Here's how the part is built. I have some questions about the finished solid (model axes, mm). A direction names the side the tool comes from. Round coordinates to 2 decimals unless told otherwise and drop trailing zeros. Loops run counter-clockwise (first coordinate to the right, second up) from the corner with the lowest first, then second, coordinate; pieces in that order, holes last. Notation, with made-up numbers: (52, 50) - (69, 50) arc R30 cw to (69, 72) - close; hole circle Ø10 at (10, -19.75). An arc over 180 degrees is marked (long way). Return JSON: item names as keys, results as strings. Group by question number.
```python
from build123d import *

# Parameters (mm, degrees)
SKETCH1_W               = 22.054431489
SKETCH1_H               = 12.5
BOSS_EXTRUDE1_DEPTH     = 38
CUT_EXTRUDE1_DEPTH      = 10
CUT_EXTRUDE1_DEPTH_BACK = 15
SKETCH2_R               = 1.5
FILLET3_R               = 2
SKETCH5_R               = 1.5
CUT_EXTRUDE4_DEPTH      = 53.86644408
SKETCH16_W              = 22.05443149
SKETCH16_H              = 2.749314183
SKETCH16_W_2            = 22.143232671
SKETCH16_H_2            = 2.765172048
CUT_EXTRUDE6_DEPTH      = 8.5
FILLET4_R               = 2
SKETCH17_W              = 18.547612126
SKETCH17_H              = 2.749314183
SKETCH17_H_2            = 2.765172048
CUT_EXTRUDE7_DEPTH      = 5
SKETCH18_W              = 23.880033653
SKETCH18_H              = 0.742090051
SKETCH18_W_2            = 23.982039935
SKETCH18_H_2            = 0.706785536
CUT_EXTRUDE8_DEPTH      = 20


with BuildPart() as part:
    # Sketch1 → Boss-Extrude1 (new body)
    with BuildSketch(Plane.XY):
        with Locations((-13.228930986, -24.070183414)):
            Rectangle(SKETCH1_W, SKETCH1_H)
    extrude(amount=BOSS_EXTRUDE1_DEPTH)

    # Sketch2 → Cut-Extrude1 (cut, two sides: drawn at the far end of the back side and taken through both)
    with BuildSketch(Plane.XZ.offset(30.320183414).offset(-CUT_EXTRUDE1_DEPTH_BACK)):
        with Locations(Location((-13.228930986, 6.5, 0), (0, 0, 90))):
            Circle(SKETCH2_R)
        with Locations(Location((-13.228930986, 31.5, 0), (0, 0, 90))):
            Circle(SKETCH2_R)
        with BuildLine():
            Line((-4.478930986, 29.25), (-2.201715242, 29.25))
            add(Edge.make_bspline(
                [(-24.256146731, 29.25), (-34.277912729, 38.417119108), (-13.227499763, 50.308047167), (7.840407292, 38.416977249), (-2.201715242, 29.25)],
                knots=[0, 0, 0, 0, 0.49986218, 1, 1, 1, 1], degree=3))
            add(Edge.make_bspline(
                [(-6.103895584, 34.329012749), (-10.720559386, 33.527203043), (-28.641384523, 40.845191705), (-24.256146731, 29.25)],
                knots=[0, 0, 0, 0, 1, 1, 1, 1], degree=3))
            ThreePointArc((-6.103895584, 34.329012749), (-4.895067543, 31.916312081), (-4.478930986, 29.25))
        make_face()
        with BuildLine():
            Line((-4.478930986, 8.75), (-2.201715242, 8.75))
            add(Edge.make_bspline(
                [(-2.201715242, 8.75), (5.39210746, 3.880294823), (-0.777052631, -4.523329032), (-17.174300591, -10.623347238), (-34.821400648, -0.026005424), (-24.256146731, 8.75)],
                knots=[0, 0, 0, 0, 0.283272691, 0.504244858, 1, 1, 1, 1], degree=3))
            add(Edge.make_bspline(
                [(-23.490579314, 0), (-24.966512963, 4.237786421), (-24.256146731, 8.75)],
                knots=[0, 0, 0, 1, 1, 1], degree=2))
            Line((-23.490579314, 0), (-13.228930986, 0))
            ThreePointArc((-13.228930986, 0), (-7.041746651, 2.562815665), (-4.478930986, 8.75))
        make_face()
    extrude(amount=CUT_EXTRUDE1_DEPTH + CUT_EXTRUDE1_DEPTH_BACK, mode=Mode.SUBTRACT)

    # Fillet3
    # the kernel refuses this fillet: 2 mm, written as the material it takes off along each edge
    with BuildSketch(Plane(origin=(-24.256146731, -17.820183414, -5.498495188), x_dir=(1, 0, 0), z_dir=(0, 0, 1))) as fillet3_piece_1:
        with BuildLine():
            CenterArc((FILLET3_R, -FILLET3_R), FILLET3_R, 90, 90)
            Line((0, -FILLET3_R), (-FILLET3_R * 0.02, -FILLET3_R))
            Line((-FILLET3_R * 0.02, -FILLET3_R), (-FILLET3_R * 0.02, FILLET3_R * 0.02))
            Line((-FILLET3_R * 0.02, FILLET3_R * 0.02), (FILLET3_R, FILLET3_R * 0.02))
            Line((FILLET3_R, FILLET3_R * 0.02), (FILLET3_R, 0))
        make_face()
    extrude(amount=44.984872581, mode=Mode.SUBTRACT)
    with BuildSketch(Plane(origin=(-24.256146731, -30.320183414, -5.498495188), x_dir=(1, 0, 0), z_dir=(0, 0, 1))) as fillet3_piece_2:
        with BuildLine():
            CenterArc((FILLET3_R, FILLET3_R), FILLET3_R, 180, 90)
            Line((0, FILLET3_R), (-FILLET3_R * 0.02, FILLET3_R))
            Line((-FILLET3_R * 0.02, FILLET3_R), (-FILLET3_R * 0.02, -FILLET3_R * 0.02))
            Line((-FILLET3_R * 0.02, -FILLET3_R * 0.02), (FILLET3_R, -FILLET3_R * 0.02))
            Line((FILLET3_R, -FILLET3_R * 0.02), (FILLET3_R, 0))
        make_face()
    extrude(amount=44.984872581, mode=Mode.SUBTRACT)
    with BuildSketch(Plane(origin=(-24.256146731, -17.374523396, 3.001504812), x_dir=(0.16676818592575765, -1.261066300243152e-15, -0.9859961319209278), z_dir=(0, -1, 0))) as fillet3_piece_3:
        with BuildLine():
            CenterArc((0.168096911, 1.999974157), FILLET3_R, 260.400032587, 9.891234523)
            Line((-0.165439461, 0.027981894), (-0.172110188, -0.011457952))
            Line((-0.172110188, -0.011457952), (-0.006670727, -0.039439845))
            Line((-0.006670727, -0.039439845), (-0.00020343, -0.039999483))
            ThreePointArc((-0.00020343, -0.039999483), (0.089132026, -0.040226606), (0.178467349, -0.039999483))
            Line((0.178467349, -0.039999483), (0.178264007, 0))
        make_face()
    extrude(amount=13.391320036, mode=Mode.SUBTRACT)
    with BuildSketch(Plane(origin=(-24.256146731, -14.125185169, 34.486377393), x_dir=(0.8125654725305003, 0, 0.5828699279009725), z_dir=(0, -1, 0))) as fillet3_piece_4:
        with BuildLine():
            CenterArc((1.058597408, -1.955531144), FILLET3_R, 77.895172565, 66.452175148)
            Line((-0.566533537, -0.789791288), (-0.599036156, -0.766476491))
            Line((-0.599036156, -0.766476491), (-0.032502619, 0.023314797))
            Line((-0.032502619, 0.023314797), (-0.009827922, 0.038773856))
            ThreePointArc((-0.009827922, 0.038773856), (0.740246051, 0.125750941), (1.486387336, 0.039110623))
            Line((1.486387336, 0.039110623), (1.477999298, 0))
        make_face()
    extrude(amount=19.88999649, mode=Mode.SUBTRACT)

    # Sketch5 → Cut-Extrude4 (cut, through all)
    with BuildSketch(Plane.XY):
        with Locations(Location((-18.011106811, -24.070183414, 0), (0, 0, 180))):
            Circle(SKETCH5_R)
        with Locations(Location((-8.446755162, -24.070183414, 0), (0, 0, 180))):
            Circle(SKETCH5_R)
    extrude(amount=CUT_EXTRUDE4_DEPTH, mode=Mode.SUBTRACT)

    # Sketch16 → Cut-Extrude6 (cut)
    with BuildSketch(Plane.XY.offset(38)):
        with Locations((-13.228930985, -20.306320009)):
            Rectangle(SKETCH16_W, SKETCH16_H)
        with Locations((-13.184530395, -27.841975748)):
            Rectangle(SKETCH16_W_2, SKETCH16_H_2)
    extrude(amount=-CUT_EXTRUDE6_DEPTH, mode=Mode.SUBTRACT)

    # Fillet4
    # the kernel refuses this fillet: 2 mm, written as the material it takes off along each edge
    with BuildSketch(Plane(origin=(-6.103895584, -22.334365667, 34.329012749), x_dir=(0.515368054600745, 0, -0.8569689424343473), z_dir=(0, 1, 0))) as fillet4_piece_1:
        with BuildLine():
            CenterArc((1.205528974, 1.993941708), FILLET4_R, 212.228268917, 62.232476225)
            Line((-0.486331325, 0.927354287), (-0.520168531, 0.906022538))
            ThreePointArc((-0.520168531, 0.906022538), (-0.25689069, 0.456334761), (-0.037300681, -0.01444504))
            Line((-0.037300681, -0.01444504), (-0.003111043, -0.039878834))
            ThreePointArc((-0.003111043, -0.039878834), (0.68054055, -0.066505026), (1.364192143, -0.039878834))
            Line((1.364192143, -0.039878834), (1.3610811, 0))
        make_face()
    extrude(amount=7.916885004, mode=Mode.SUBTRACT)
    with BuildSketch(Plane(origin=(-6.103895584, -29.862092474, 34.329012749), x_dir=(0.515368054600745, 0, -0.8569689424343473), z_dir=(0, 1, 0))) as fillet4_piece_2:
        with BuildLine():
            CenterArc((1.205528974, 1.993941708), FILLET4_R, 212.228268917, 62.232476225)
            Line((-0.486331325, 0.927354287), (-0.520168531, 0.906022538))
            ThreePointArc((-0.520168531, 0.906022538), (-0.25689069, 0.456334761), (-0.037300681, -0.01444504))
            Line((-0.037300681, -0.01444504), (-0.003111043, -0.039878834))
            ThreePointArc((-0.003111043, -0.039878834), (0.68054055, -0.066505026), (1.364192143, -0.039878834))
            Line((1.364192143, -0.039878834), (1.3610811, 0))
        make_face()
    extrude(amount=11.583818124, mode=Mode.SUBTRACT)
    with BuildSketch(Plane(origin=(-6.103895584, -33.722886164, 34.329012749), x_dir=(0.515368054600745, 0, -0.8569689424343473), z_dir=(0, 1, 0))) as fillet4_piece_3:
        with BuildLine():
            CenterArc((1.205528974, 1.993941708), FILLET4_R, 212.228268917, 62.232476225)
            Line((-0.486331325, 0.927354287), (-0.520168531, 0.906022538))
            ThreePointArc((-0.520168531, 0.906022538), (-0.25689069, 0.456334761), (-0.037300681, -0.01444504))
            Line((-0.037300681, -0.01444504), (-0.003111043, -0.039878834))
            ThreePointArc((-0.003111043, -0.039878834), (0.68054055, -0.066505026), (1.364192143, -0.039878834))
            Line((1.364192143, -0.039878834), (1.3610811, 0))
        make_face()
    extrude(amount=7.901027143, mode=Mode.SUBTRACT)

    # Sketch17 → Cut-Extrude7 (cut)
    with BuildSketch(Plane.XY.offset(29.5)):
        with Locations((-13.756309207, -20.306320009)):
            Rectangle(SKETCH17_W, SKETCH17_H)
        with Locations((-13.756309207, -27.841975748)):
            Rectangle(SKETCH17_W, SKETCH17_H_2)
    extrude(amount=-CUT_EXTRUDE7_DEPTH, mode=Mode.SUBTRACT)

    # Sketch18 → Cut-Extrude8 (cut)
    with BuildSketch(Plane.XY):
        with Locations((-13.859477608, -30.474932984)):
            Rectangle(SKETCH18_W, SKETCH18_H)
        with Locations((-13.808474467, -17.715166293)):
            Rectangle(SKETCH18_W_2, SKETCH18_H_2)
    extrude(amount=CUT_EXTRUDE8_DEPTH, mode=Mode.SUBTRACT)


solid = part.part
```
Q1. Please list where these lines run through material, in increasing order: line 1 (Y direction, x = -21.25, z = 34.5); line 2 (X direction, y = -24.25, z = 23.5); line 3 (X direction, y = -23.75, z = 31.5).
Q2. Imagine slicing it at D-D, the plane y = -26. Give the number of separate pieces and of enclosed holes in the cut face, and give its area (3 significant figures).
Q3. Will these pins go through, and if not, where does the flat tip stop? pin 1 Ø4 at (x, y) = (-18.01, -24.07) entering from +Z; pin 2 Ø1.5 at (x, z) = (-17, 18) entering from +Y; pin 3 Ø1.8 at (x, y) = (-3, -24.5) entering from -Z; pin 4 Ø2.5 at (x, z) = (-13.23, 31.5) entering from -Y.
Q4. If we mould it in two halves opening along Y, with no side actions, what happens to faces 1 (the flat face through (-13, -30.104, 10)), 2 (the flat face through (-24, -20, 29.5)), 3 (the cylindrical face through (-6.135, -18.384, 33.966)), 4 (the flat face through (-23.03, -28, 27))? For each: +Y half, -Y half, draft (parallel to the pull), parting line (faces both ways), or undercut.
Q5. For faces 5 (the flat face through (-23.03, -20, 27)), 6 (the flat face through (-2.202, -24, 19)), 7 (the cylindrical face through (-23.92, -24.037, 34.624)), 8 (the flat face through (-13, -18.069, 10)), 9 (the flat face through (-24, -28, 29.5)), which set-ups out of +Z, -Z, +X, -X, +Y, -Y let a thin tool reach every point of the face, with its end or its side?
Q6. Imagine slicing it at C-C, the plane z = 12. List the corners of the cut face in (x, y) for me.
Q7. Imagine slicing it at A-A, the plane z = 6. List the corners of the cut face in (x, y) for me, and give its area (3 significant figures).
Q8. Imagine slicing it at B-B, the plane z = 31. List the corners of the cut face in (x, y) for me.
Output values:
{
 "1": {"line 1": "y = -30.32 to -29.22, -26.46 to -21.68, -18.93 to -17.82", "line 2": "x = -24.26 to -19.5, -16.52 to -9.94, -6.96 to -2.2", "line 3": "x = -24.26 to -19.48, -16.55 to -14.73, -11.73 to -9.91, -6.98 to -4.77"},
 "2": {"separate pieces": "1", "enclosed holes": "2", "area": "706 mm^2"},
 "3": {"pin 1": "stops at z = 35.88", "pin 2": "stops at y = -18.07", "pin 3": "stops at z = 8.75", "pin 4": "passes through"},
 "4": {"face 1": "-Y half", "face 2": "undercut", "face 3": "draft", "face 4": "undercut"},
 "5": {"face 5": "+Z", "face 6": "+Z, -Z, +X, +Y, -Y", "face 7": "+Z, -X, +Y, -Y", "face 8": "-Z, +X, -X, +Y", "face 9": "+Z, +X, -X"},
 "6": {"outline": "(-24.26, -28.32) arc R2 ccw to (-23.16, -30.1) - (-2.2, -30.1) - (-2.2, -18.07) - (-23.22, -18.07) arc R2 ccw to (-24.26, -19.82) - close; hole circle Ø3 at (-18.01, -24.07); hole circle Ø3 at (-8.45, -24.07)"},
 "7": {"outline": "(-24.26, -28.32) arc R2 ccw to (-23.16, -30.1) - (-14.64, -30.1) - (-14.64, -18.07) - (-23.22, -18.07) arc R2 ccw to (-24.26, -19.82) - close; (-11.81, -30.1) - (-4.92, -30.1) - (-4.92, -18.07) - (-11.81, -18.07) - close; hole circle Ø3 at (-18.01, -24.07); hole circle Ø3 at (-8.45, -24.07)", "area": "183 mm^2"},
 "8": {"outline": "(-24.26, -26.46) - (-14.64, -26.46) - (-14.64, -21.68) - (-24.26, -21.68) - close; (-24.05, -18.93) - (-14.64, -18.93) - (-14.64, -17.82) - (-22.26, -17.82) arc R2 ccw to start; (-24.04, -29.22) arc R2 ccw to (-22.26, -30.32) - (-14.64, -30.32) - (-14.64, -29.22) - close; (-11.81, -30.32) - (-4.66, -30.32) - (-4.66, -29.22) - (-11.81, -29.22) - close; (-11.81, -26.46) - (-4.66, -26.46) - (-4.66, -21.68) - (-11.81, -21.68) - close; (-11.81, -18.93) - (-4.66, -18.93) - (-4.66, -17.82) - (-11.81, -17.82) - close; hole circle Ø3 at (-18.01, -24.07); hole circle Ø3 at (-8.45, -24.07)"}
}
